Source: CAD feature listing. Evaluate the final solid. Frame: model axes, mm. Coordinates: 2 decimals unless noted, no trailing zeros. Loops run counter-clockwise (first coordinate to the right, second up) from the corner with the lowest first, then second, coordinate; pieces in that order, holes last.
Item 1: Section query D-D, the plane y = 13.5. Return the cut outline in (x, z), then the cut area to 3 significant figures.
Item 2: Section query A-A, the plane z = 1.25. Return the cut outline in (x, y) (3 decimals).
Item 3: Section query B-B, the plane y = -3. Return the cut outline in (x, z).
Item 4: Pin query (flat end, axial travel): pin 1 Ø1 at (y, z) = (12, 5) entering from +X; pin 2 Ø3 at (y, z) = (14, 2.5) entering from -X. Return the tip coordinate at first contact, or that it passes through.
Item 5: Section query C-C, the plane x = -33. Return the cut outline in (y, z).
Item 6: Line query: probe 1 along X at (y, z) = (10, 2.5); probe 2 along X at (y, z) = (-1.5, 0.5); probe 3 along Y at (x, z) = (-28, 3.75). Output: solid intervals per line, ascending.
```python
from build123d import *

# Parameters (mm, degrees)
F1_DEPTH = 6.604


with BuildPart() as f1:
    # F0 (on Top) → F1 (new body)
    with BuildSketch(Plane.XY):
        with BuildLine():
            Line((-35, 5.9436), (-35, 25.5))
            ThreePointArc((-35, 25.5), (-60.5, 0), (-35, -25.5))
            Line((-35, -25.5), (-35, -5.9436))
            ThreePointArc((-35, -5.9436), (-40.49117, -2.274517), (-39.20276, 4.20276))
            ThreePointArc((-39.20276, 4.20276), (-37.274517, 5.49117), (-35, 5.9436))
        make_face()
        with BuildLine():
            ThreePointArc((-41.338835, -8.839565), (-45.606602, -10.607332), (-43.838835, -6.339565))
            ThreePointArc((-43.838835, -6.339565), (-42.071068, -7.071798), (-41.338835, -8.839565))
        make_face(mode=Mode.SUBTRACT)
        with BuildLine():
            ThreePointArc((-41.338835, 8.838835), (-41.529136, 7.882126), (-42.071068, 7.071068))
            ThreePointArc((-42.071068, 7.071068), (-42.882126, 6.529136), (-43.838835, 6.338835))
            ThreePointArc((-43.838835, 6.338835), (-45.606602, 10.606602), (-41.338835, 8.838835))
        make_face(mode=Mode.SUBTRACT)
        with BuildLine():
            Line((35, 9.525), (35, 25.5))
            Line((35, 25.5), (-35, 25.5))
            Line((-35, 25.5), (-35, 5.9436))
            ThreePointArc((-35, 5.9436), (-30.79724, 4.20276), (-29.0564, 0))
            ThreePointArc((-29.0564, 0), (-29.50883, -2.274517), (-30.79724, -4.20276))
            ThreePointArc((-30.79724, -4.20276), (-32.725483, -5.49117), (-35, -5.9436))
            Line((-35, -5.9436), (-35, -25.5))
            Line((-35, -25.5), (35, -25.5))
            Line((35, -25.5), (35, -9.525))
            ThreePointArc((35, -9.525), (25.475, 0), (35, 9.525))
        make_face()
        with BuildLine():
            ThreePointArc((-23.663428, -8.836572), (-27.120137, -11.146271), (-27.931195, -7.068805))
            ThreePointArc((-27.931195, -7.068805), (-27.120137, -6.526873), (-26.163428, -6.336572))
            ThreePointArc((-26.163428, -6.336572), (-24.395661, -7.068805), (-23.663428, -8.836572))
        make_face(mode=Mode.SUBTRACT)
        with BuildLine():
            ThreePointArc((-23.663428, 8.841828), (-24.395661, 7.074061), (-26.163428, 6.341828))
            ThreePointArc((-26.163428, 6.341828), (-27.931195, 10.609595), (-23.663428, 8.841828))
        make_face(mode=Mode.SUBTRACT)
        with BuildLine():
            ThreePointArc((35, -25.5), (60.5, 0), (35, 25.5))
            Line((35, 25.5), (35, 9.525))
            ThreePointArc((35, 9.525), (41.735192, 6.735192), (44.525, 0))
            ThreePointArc((44.525, 0), (41.735192, -6.735192), (35, -9.525))
            Line((35, -9.525), (35, -25.5))
        make_face()
    extrude(amount=F1_DEPTH)


solid = f1.part
```
Verdict:
1. outline: (-56.63, 0) - (56.63, 0) - (56.63, 6.6) - (-56.63, 6.6) - close
1. area: 748 mm2
2. outline: (-35, -25.5) - (35, -25.5) arc R25.5 ccw to (35, 25.5) - (-35, 25.5) arc R25.5 ccw to start; hole circle Ø5 at (-43.839, -8.84); hole (-43.839, 6.339) arc R2.5 ccw to (-42.071, 7.071) arc R2.5 ccw to (-41.339, 8.839) arc R2.5 ccw (long way) to start; hole (-39.203, 4.203) arc R5.944 ccw to (-35, -5.944) arc R5.944 ccw to (-30.797, -4.203) arc R5.944 ccw to (-29.056, 0) arc R5.944 ccw to (-35, 5.944) arc R5.944 ccw to start; hole circle Ø5 at (-26.163, 8.842); hole (-27.931, -7.069) arc R2.5 ccw (long way) to (-26.163, -6.337) arc R2.5 ccw to start; hole circle Ø19.05 at (35, 0)
3. outline: (-60.32, 0) - (-40.13, 0) - (-40.13, 6.6) - (-60.32, 6.6) - close; (-29.87, 0) - (25.96, 0) - (25.96, 6.6) - (-29.87, 6.6) - close; (44.04, 0) - (60.32, 0) - (60.32, 6.6) - (44.04, 6.6) - close
4. pin 1: stops at x = 57.76
4. pin 2: stops at x = -57.23
5. outline: (-25.5, 0) - (-5.6, 0) - (-5.6, 6.6) - (-25.5, 6.6) - close; (5.6, 0) - (25.5, 0) - (25.5, 6.6) - (5.6, 6.6) - close
6. probe 1: x = -58.46 to -46.05, -41.62 to -28.38, -23.95 to 58.46
6. probe 2: x = -60.46 to -40.75, -29.25 to 25.59, 44.41 to 60.46
6. probe 3: y = -25.5 to -10.53, -7.14 to 7.15, 10.54 to 25.5
